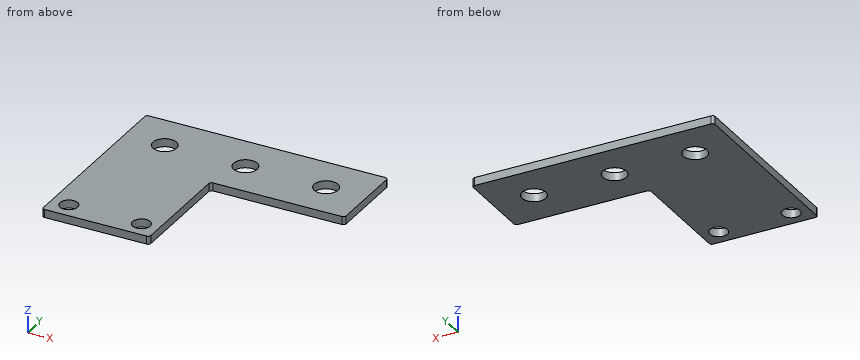
from build123d import *

# Parameters (mm, degrees)
SKETCH_1_R      = 3.3
SKETCH_1_R_2    = 4.4
EXTRUDE_1_DEPTH = 3
FILLET_1_R      = 1


with BuildPart() as part:
    # 草图1 → 凸台-拉伸1 (new body)
    with BuildSketch(Plane.XY):
        Polygon((0, 0), (0, -72), (40, -72), (40, -30), (90, -30), (90, 0), align=None)
        with Locations((33.5, -65.5)):
            Circle(SKETCH_1_R, mode=Mode.SUBTRACT)
        with Locations((6.5, -65.5)):
            Circle(SKETCH_1_R, mode=Mode.SUBTRACT)
        with Locations((45, -15)):
            Circle(SKETCH_1_R_2, mode=Mode.SUBTRACT)
        with Locations((75, -15)):
            Circle(SKETCH_1_R_2, mode=Mode.SUBTRACT)
        with Locations((15, -15)):
            Circle(SKETCH_1_R_2, mode=Mode.SUBTRACT)
    extrude(amount=EXTRUDE_1_DEPTH)

    # 圆角1
    fillet_1_edges = [part.edges().sort_by_distance(p)[0] for p in [
        (90, 0, 1.5),
        (90, -30, 1.5),
        (40, -30, 1.5),
        (40, -72, 1.5),
        (0, -72, 1.5),
        (0, 0, 1.5),
    ]]
    fillet(fillet_1_edges, radius=FILLET_1_R)


solid = part.part
Verification items for the finished model (mm, model axes). Round coordinates to 2 decimals unless told otherwise and drop trailing zeros. Write each loop counter-clockwise with the first axis right and the second up, starting at its lowest first coordinate (ties: lowest second). Pieces come first, ordered by that corner, then holes.
(1) Material ranges on line 1 (Y direction, x = 6.5, z = 1.2); line 2 (Y direction, x = 75, z = 1.2); line 3 (X direction, y = -14, z = 1.3), recorded low to high.
Returned:
line 1: y = -72 to -68.8, -62.2 to 0
line 2: y = -30 to -19.4, -10.6 to 0
line 3: x = 0 to 10.72, 19.28 to 40.72, 49.28 to 70.72, 79.28 to 90
(2) Section check A-A (y = -15). Enter the section's corners in (x, z).
Returned:
outline: (0, 0) - (10.6, 0) - (10.6, 3) - (0, 3) - close; (19.4, 0) - (40.6, 0) - (40.6, 3) - (19.4, 3) - close; (49.4, 0) - (70.6, 0) - (70.6, 3) - (49.4, 3) - close; (79.4, 0) - (90, 0) - (90, 3) - (79.4, 3) - close
(3) Section check D-D (y = -65.5). Enter the section's corners in (x, z), plus the area to 3 significant figures.
Returned:
outline: (0, 0) - (3.2, 0) - (3.2, 3) - (0, 3) - close; (9.8, 0) - (30.2, 0) - (30.2, 3) - (9.8, 3) - close; (36.8, 0) - (40, 0) - (40, 3) - (36.8, 3) - close
area: 80.4 mm2
(4) Section check B-B (x = 75). Enter the section's corners in (y, z), plus the area to 3 significant figures.
Returned:
outline: (-30, 0) - (-19.4, 0) - (-19.4, 3) - (-30, 3) - close; (-10.6, 0) - (0, 0) - (0, 3) - (-10.6, 3) - close
area: 63.6 mm2
(5) Section check C-C (z = 1). Enter the section's corners in (x, y), plus the area to 3 significant figures.
Returned:
outline: (0, -71) arc R1 ccw to (1, -72) - (39, -72) arc R1 ccw to (40, -71) - (40, -31) arc R1 cw to (41, -30) - (89, -30) arc R1 ccw to (90, -29) - (90, -1) arc R1 ccw to (89, 0) - (1, 0) arc R1 ccw to (0, -1) - close; hole circle Ø6.6 at (6.5, -65.5); hole circle Ø8.8 at (15, -15); hole circle Ø6.6 at (33.5, -65.5); hole circle Ø8.8 at (45, -15); hole circle Ø8.8 at (75, -15)
area: 4,130 mm2
(6) Depth check by flat-ended pin: pin 1 Ø1 at (y, z) = (-59.5, 0.5) entering from +X. Enter the tip coordinate at first touch or a pass-through.
Returned:
pin 1: stops at x = 40
